Here's the drawing with two shaded views (mm, measured from the low corner). I have some questions. A direction names the side the tool comes from. Round coordinates to 2 decimals unless told otherwise and drop trailing zeros. Loops run counter-clockwise (first coordinate to the right, second up) from the corner with the lowest first, then second, coordinate; pieces in that order, holes last. Notation, with made-up numbers: M 66.5,12.25 L 110.5,12.25 A16 ccw 110.5,34.25 Z; hole C 28.5,61.5 d5. An arc over 180 degrees is marked long. Write each question's results on one line, items separated by ' | '. Start each with the question number.
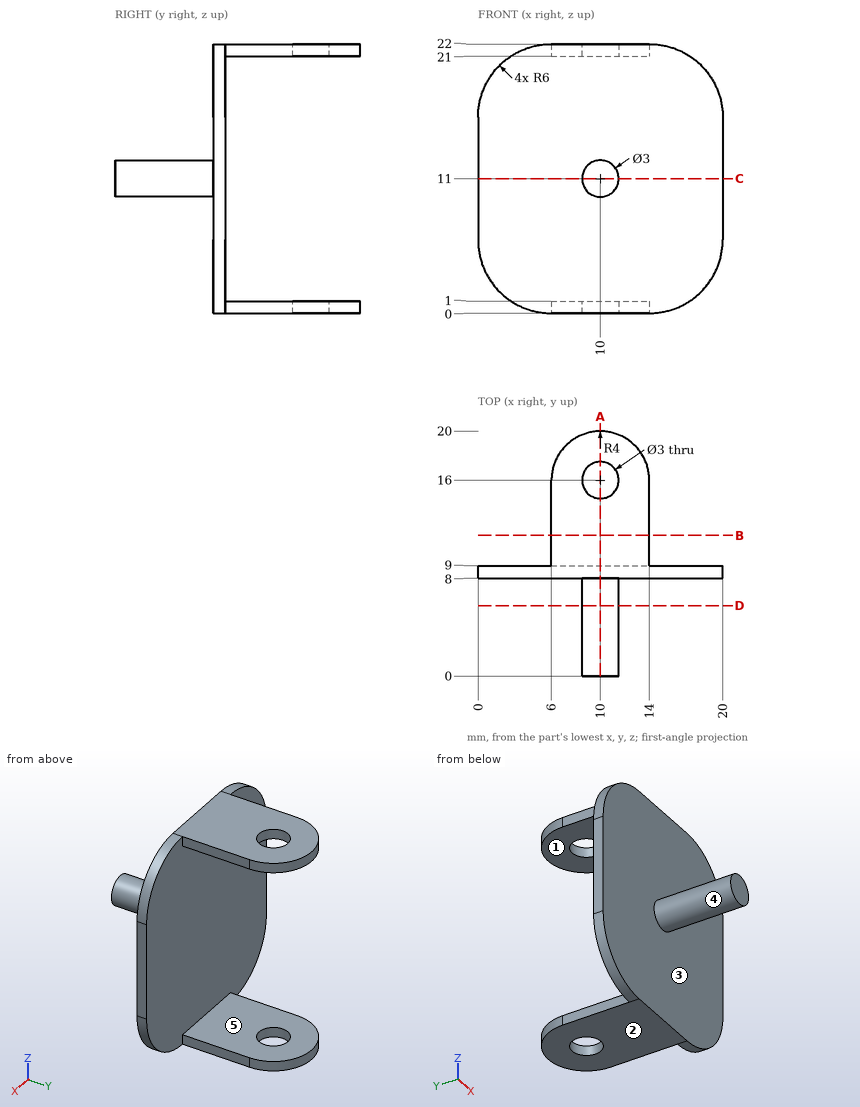
Item 1: If we mould it in two halves opening along Z, with no side actions, what happens to the marked faces 3, 4 and 5? For each: released by +Z, released by -Z, zero draft, split by the parting line, or undercut.
Item 2: I need wall thicknesses on L1, parallel to Y at x = 10, z = 0.75; L2, parallel to Z at x = 12, y = 15.75; L3, parallel to X at y = 13, z = 21.25. Which ranges of each line are inside material? Lowest first, please.
Item 3: If we section it at D-D on y = 5.75: Please give me the cut outline in (x, z), and give its area (3 significant figures).
Item 4: Which directions (+Z, -Z, +X, -X, +Y, -Y) give clear straight access to the entire face, cutting with the end or side of a thin tool? Please do the marked faces 1 and 2.
Item 5: If we section it at A-A on x = 10: Please give me the cut outline in (y, z).
Item 6: I'm going to push flat-ended pins straight in: pin 1 (0.5 mm diameter, centred on y = 12.5, z = 0.5, fed in from +X); pin 2 (1 mm diameter, centred on x = 2.5, z = 8.5, fed in from -Y); pin 3 (5 mm diameter, centred on y = 5, z = 12, fed in from -X). Where does each tip first touch, or does it pass through?
Item 7: If we section it at B-B on y = 11.5: Please give me the cut outline in (x, z), and give its area (3 significant figures).
Item 8: If we section it at C-C on z = 11: Please give me the cut outline in (x, y), and give its area (3 significant figures).
Numbers:
1) face 3: zero draft | face 4: split by the parting line | face 5: undercut
2) L1: 8 to 14.5, 17.5 to 20 | L2: 0 to 1, 21 to 22 | L3: 6 to 14
3) outline: C 10,11 d3 | area: 7.07 mm²
4) face 1: +X, -X, +Y | face 2: -Z, +X, -X, +Y, -Y
5) outline: M 0,9.5 L 8,9.5 L 8,0 L 14.5,0 L 14.5,1 L 9,1 L 9,21 L 14.5,21 L 14.5,22 L 8,22 L 8,12.5 L 0,12.5 Z; M 17.5,0 L 20,0 L 20,1 L 17.5,1 Z; M 17.5,21 L 20,21 L 20,22 L 17.5,22 Z
6) pin 1: x = 14 | pin 2: y = 8 | pin 3: x = 8.5
7) outline: M 6,0 L 14,0 L 14,1 L 6,1 Z; M 6,21 L 14,21 L 14,22 L 6,22 Z | area: 16.0 mm²
8) outline: M 0,8 L 8.5,8 L 8.5,0 L 11.5,0 L 11.5,8 L 20,8 L 20,9 L 0,9 Z | area: 44.0 mm²
